```python
from build123d import *

# Parameters (mm, degrees)
SKETCH001_R  = 12
PAD001_DEPTH = 8
SKETCH_R     = 12
SKETCH_R_2   = 3
PAD_DEPTH    = 4
CHAMFER_SIZE = 1


with BuildPart() as part:
    # Sketch001 → Pad001 (new body)
    with BuildSketch(Plane.XY.offset(4)):
        Circle(SKETCH001_R)
        Polygon((4.907477, -8.5), (9.814955, 0), (4.907477, 8.5), (-4.907477, 8.5), (-9.814955, 0), (-4.907477, -8.5), align=None, mode=Mode.SUBTRACT)
    extrude(amount=PAD001_DEPTH)

    # Sketch (on Face8 of Pad001) → Pad (join)
    with BuildSketch(Plane(origin=(0, 0, 4), x_dir=(1, 0, 0), z_dir=(0, 0, -1))):
        Circle(SKETCH_R)
        Circle(SKETCH_R_2, mode=Mode.SUBTRACT)
    extrude(amount=PAD_DEPTH)

    # Chamfer
    chamfer_edges = [part.edges().sort_by_distance(p)[0] for p in [
        (-7.361216, -4.25, 12),
        (-7.361216, 4.25, 12),
        (0, 8.5, 12),
        (7.361216, 4.25, 12),
        (0, -8.5, 12),
        (7.361216, -4.25, 12),
    ]]
    chamfer(chamfer_edges, length=CHAMFER_SIZE)


solid = part.part
```
Source: CAD feature listing. Evaluate the final solid. Frame: model axes, mm. A direction names the side the tool comes from. Coordinates: 2 decimals unless noted, no trailing zeros. Loops run counter-clockwise (first coordinate to the right, second up) from the corner with the lowest first, then second, coordinate; pieces in that order, holes last. Notation, with made-up numbers: M -2,28.25 L 39,28.25 A27 ccw 39,52.25 Z; hole C 86,84 d11. An arc over 180 degrees is marked long. Use a Markdown table: item, result. Add a question column.
Q1. Section query A-A, the plane x = 0. Return loops of the section in (y, z), and give its area (3 significant figures).
Q2. Section query B-B, the plane z = 5.5. Return loops of the section in (x, y), and give its area (3 significant figures).
Q3. Access query for faces 4 (the flat face through (-0.1, -9, 11.5)), 5 (the cylindrical face through (-3, 0, 2)). Directions: +Z, -Z, +X, -X, +Y, -Y. A direction counts if a zero-diameter tool reaches every point of the face in a straight line with its end or side. Return the directions, or none.
Q4. Material intervals for L1, parallel to X at y = 0, z = 1.3; L2, parallel to Z at x = 6.5, y = 2.5, sorted ascending.
Q5. Draft query along X for faces 1 (the flat face through (-8.1, -5.3, 12)), 2 (the flat face through (7.827, 4.43, 11.493)), 3 (the cylindrical face through (-11.99, -0.53, 6.08)). Return one class per face: pulls with the +X half, pulls with the -X half, needs draft (parallel to the pull), parting line crosses it, or undercut.
Q6. First-contact query: pin 1 (1.5 mm diameter, centred on x = 3, z = 9, fed in from +Y); pin 2 (8.5 mm diameter, centred on x = -2.5, y = -1.5, fed in from +Z); pin 3 (2 mm diameter, centred on y = -2, z = 9, fed in from -X). Flat tips, straight axial feed; report the tip coordinate or a pass-through.
Q7. Section query C-C, the plane y = 1.5. Return loops of the section in (x, z).
Q8. Section query D-D, the plane x = -9.5. Return loops of the section in (y, z), and give its area (3 significant figures).
Result:
| question | item | result |
|---|---|---|
| 1 | outline | M -12,0 L -3,0 L -3,4 L -8.5,4 L -8.5,11 L -9.5,12 L -12,12 Z; M 3,0 L 12,0 L 12,12 L 9.5,12 L 8.5,11 L 8.5,4 L 3,4 Z |
| 1 | area | 127 mm2 |
| 2 | outline | C 0,0 d24; hole M -9.81,0 L -4.91,-8.5 L 4.91,-8.5 L 9.81,0 L 4.91,8.5 L -4.91,8.5 Z |
| 2 | area | 202 mm2 |
| 3 | face 4 | +Z |
| 3 | face 5 | +Z, -Z |
| 4 | L1 | x = -12 to -3, 3 to 12 |
| 4 | L2 | z = 0 to 4 |
| 5 | face 1 | needs draft |
| 5 | face 2 | undercut |
| 5 | face 3 | parting line crosses it |
| 6 | pin 1 | stops at y = 11.79 |
| 6 | pin 2 | stops at z = 4 |
| 6 | pin 3 | stops at x = -11.96 |
| 7 | outline | M -11.91,0 L -2.6,0 L -2.6,4 L -8.95,4 L -8.95,11 L -10.1,12 L -11.91,12 Z; M 2.6,0 L 11.91,0 L 11.91,12 L 10.1,12 L 8.95,11 L 8.95,4 L 2.6,4 Z |
| 8 | outline | M -7.33,0 L 7.33,0 L 7.33,12 L 2.55,12 L 0.55,11 L 0.55,4 L -0.55,4 L -0.55,11 L -2.55,12 L -7.33,12 Z |
| 8 | area | 165 mm2 |
